```python
from build123d import *

# Parameters (mm, degrees)
BOSS_EXTRUDE1_DEPTH = 5
CUT_EXTRUDE1_DEPTH  = 6


with BuildPart() as part:
    # Sketch1 → Boss-Extrude1 (new body)
    with BuildSketch(Plane.XY):
        Polygon((-75, 50), (-70, 50), (-70, 55), (-54.25, 55), (-54.25, 50), (-38.9375, 50), (-38.9375, 55), (-23.1875, 55), (-23.1875, 50), (-7.875, 50), (-7.875, 55), (7.875, 55), (7.875, 50), (23.1875, 50), (23.1875, 55), (38.9375, 55), (38.9375, 50), (54.25, 50), (54.25, 55), (70, 55), (70, 50), (75, 50), (75, 45), (80, 45), (80, 27), (75, 27), (75, 9), (80, 9), (80, -9), (75, -9), (75, -27), (80, -27), (80, -45), (75, -45), (75, -50), (70, -50), (70, -55), (54.25, -55), (54.25, -50), (38.9375, -50), (38.9375, -55), (23.1875, -55), (23.1875, -50), (7.875, -50), (7.875, -55), (-7.875, -55), (-7.875, -50), (-23.1875, -50), (-23.1875, -55), (-38.9375, -55), (-38.9375, -50), (-54.25, -50), (-54.25, -55), (-70, -55), (-70, -50), (-75, -50), (-75, -45), (-80, -45), (-80, -27), (-75, -27), (-75, -9), (-80, -9), (-80, 9), (-75, 9), (-75, 27), (-80, 27), (-80, 45), (-75, 45), align=None)
    extrude(amount=BOSS_EXTRUDE1_DEPTH)

    # Sketch2 → Cut-Extrude1 (cut, through all)
    with BuildSketch(Plane(origin=(0, 0, 0), x_dir=(-1, 0, 0), z_dir=(0, 0, -1))):
        Polygon((-47, 45), (43, 45), (43, 39), (69, 39), (69, 5), (43, 5), (43, -45), (-47, -45), align=None)
    extrude(amount=-CUT_EXTRUDE1_DEPTH, mode=Mode.SUBTRACT)


solid = part.part
```
Read the model definition and answer for the solid it produces. Units are mm, in the model's axes. A direction names the side the tool comes from. Round coordinates to 2 decimals unless told otherwise and drop trailing zeros. Write each loop counter-clockwise with the first axis right and the second up, starting at its lowest first coordinate (ties: lowest second). Pieces come first, ordered by that corner, then holes. Notation, with made-up numbers: M 88.5,88.5 L 113.5,88.5 A33 ccw 113.5,120.5 Z; hole C 1,60 d2. An arc over 180 degrees is marked long. One line per item, written item: value.
Q1. Straight lines are drawn through the part: line 1 (Y direction, x = -55.5, z = 4.35); line 2 (X direction, y = 41.5, z = 0.9); line 3 (Y direction, x = -41.5, z = 1.4). For each, find the intervals that lie inside material, in ascending order. Write a range as [from, to].
Data:
line 1: [-55, 5], [39, 55]
line 2: [-80, -43], [47, 80]
line 3: [-50, -45], [45, 50]
Q2. Find section A-A on y = -31.5. Write down the section's boundary in (x, z).
Data:
outline: M -80,0 L -43,0 L -43,5 L -80,5 Z; M 47,0 L 80,0 L 80,5 L 47,5 Z
Q3. Which of the six approach directions +Z, -Z, +X, -X, +Y, -Y give full straight-line access (tool end or side, diameter ignored) to faces 4 (the flat face through (7.875, 53, 2)), 5 (the flat face through (-70, -53, 2)), 6 (the flat face through (38.938, -52, 2))?
Data:
face 4: +Z, -Z, +Y
face 5: +Z, -Z, -X, -Y
face 6: +Z, -Z, -Y
Q4. Flat-ended cylindrical pins translate along their axes: pin 1 Ø1.5 at (x, z) = (78.5, 3.5) entering from +Y; pin 2 Ø2.5 at (x, z) = (77.5, 1.5) entering from -Y; pin 3 Ø1.5 at (x, z) = (14, 3.5) entering from -Y. Find the tip coordinate at first contact, or state that the pin passes through.
Data:
pin 1: y = 45
pin 2: y = -45
pin 3: y = -50
Q5. For a pull along Y with two mould halves and no side action, classify faces 1 (the flat face through (-62, 55, 2)), 2 (the flat face through (-75, 18, 2)), 3 (the flat face through (23.188, 52, 2)) as +Y half, -Y half, draft (parallel to the pull), parting line (faces both ways), or undercut.
Data:
face 1: +Y half
face 2: undercut
face 3: draft
Q6. Find section B-B on x = 26. Write down the section's boundary in (y, z).
Data:
outline: M -55,0 L -45,0 L -45,5 L -55,5 Z; M 45,0 L 55,0 L 55,5 L 45,5 Z
